Source: CAD feature listing. Evaluate the final solid. Frame: model axes, mm. Face numbers are marked on the shaded views. A direction names the side the tool comes from. Coordinates: 2 decimals unless noted, no trailing zeros. Write each loop counter-clockwise with the first axis right and the second up, starting at its lowest first coordinate (ties: lowest second). Pieces come first, ordered by that corner, then holes. Notation, with made-up numbers: M 83.5,0 L 126.5,0 A17 ccw 126.5,12 Z; hole C 74.25,-19.75 d2. An arc over 180 degrees is marked long. One line per item, written item: value. Start each with the question number.
Item 1: Cut plane A-A, the plane z = -98.5. Output: boundary loops of the cut face in (x, y), then the cut area to 3 significant figures.
Item 2: Ray query, L1, parallel to X at y = 19.5, z = -37; L2, parallel to Z at x = 19, y = 0.5; L3, parallel to Z at x = 75.5, y = -14. Return the intervals inside material, ascending. Write a range as from..to.
Item 3: Cut plane B-B, the plane y = 0. Output: boundary loops of the cut face in (x, z), then the cut area to 3 significant figures.
Item 4: Cut plane D-D, the plane z = 0. Output: boundary loops of the cut face in (x, y).
Item 5: Cut plane C-C, the plane x = 140.5. Output: boundary loops of the cut face in (y, z), then the cut area to 3 significant figures.
Item 6: Mould query, pull axis X, two halves, no side actions, for the marked faces 1, 2 and 3. Classes: released by +X, released by -X, zero draft, split by the parting line, or undercut.
Item 7: Set-up query: the marked faces 4, 5, 6, 7 and 8. Return all of +Z, -Z, +X, -X, +Y, -Y with unobstructed straight access to the full face (end or side cutting, diameter ignored); none if empty.
Item 8: Pin query (flat end, axial travel): P1, Ø12, axis at y = -7, z = -57, coming from the +X side; P2, Ø4.5, axis at y = -5, z = -223, coming from the +X side; P3, Ø10, axis at x = -26, z = -142, coming from the -Y side. Return the tip coordinate at first contact, or that it passes through.
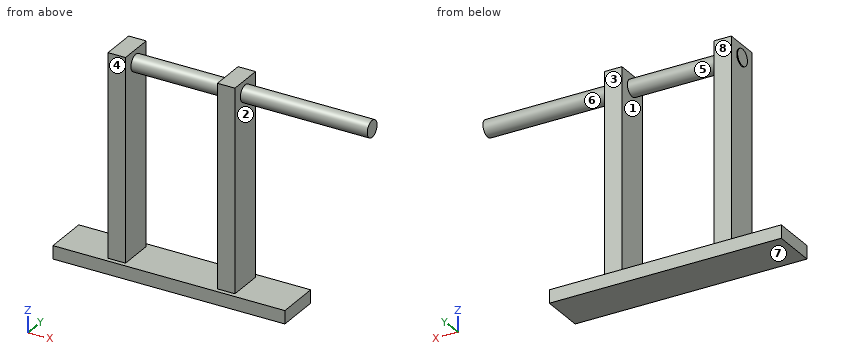
```python
from build123d import *

# Parameters (mm, degrees)
F0_R      = 9.5
F1_DEPTH  = 40
F2_R      = 9.5
F3_DEPTH  = 70
F4_R      = 9.5
F5_DEPTH  = 180
F6_W      = 20
F6_H      = 20
F7_DEPTH  = 15
F8_W      = 20
F8_H      = 10
F9_DEPTH  = 215
F11_DEPTH = 15
F12_DEPTH = 15
F13_DEPTH = 215
F15_DEPTH = 215
F16_W     = 20
F16_H     = 7.5
F17_DEPTH = 20
F18_DEPTH = 25
F19_DEPTH = 25
F20_R     = 9.5
F21_DEPTH = 1


with BuildPart() as f1:
    # F0 (on Right) → F1 (new body)
    with BuildSketch(Plane.YZ):
        Circle(F0_R)
    extrude(amount=-F1_DEPTH)

    # F2 (on face) → F3 (join)
    with BuildSketch(Plane.YZ):
        Circle(F2_R)
    extrude(amount=F3_DEPTH)

    # F4 (on face) → F5 (join)
    with BuildSketch(Plane.YZ.offset(70)):
        Circle(F4_R)
    extrude(amount=F5_DEPTH)

    # F6 (on Top) → F7 (join)
    with BuildSketch(Plane.XY):
        with Locations((-30, -10)):
            Rectangle(F6_W, F6_H)
        with Locations((-30, 10)):
            Rectangle(F6_W, F6_H)
    extrude(amount=F7_DEPTH)

    # F8 (on Top) → F9 (join)
    with BuildSketch(Plane.XY):
        with Locations((-30, -5)):
            Rectangle(F8_W, F8_H)
        with Locations((-30, 5)):
            Rectangle(F8_W, F8_H)
        with Locations((-30, -15)):
            Rectangle(F8_W, F8_H)
        with Locations((-30, 15)):
            Rectangle(F8_W, F8_H)
    extrude(amount=-F9_DEPTH)

    # F10 (on Top) → F11 (join)
    with BuildSketch(Plane.XY):
        Polygon((85, 10), (85, 0), (85, -10), (85, -20), (105, -20), (105, 20), (85, 20), align=None)
    extrude(amount=F11_DEPTH)

    # F6 (on Top) → F12 (join)
    with BuildSketch(Plane.XY):
        with Locations((-30, -10)):
            Rectangle(F6_W, F6_H)
        with Locations((-30, 10)):
            Rectangle(F6_W, F6_H)
    extrude(amount=F12_DEPTH)

    # F8 (on Top) → F13 (join)
    with BuildSketch(Plane.XY):
        with Locations((-30, -5)):
            Rectangle(F8_W, F8_H)
        with Locations((-30, 5)):
            Rectangle(F8_W, F8_H)
        with Locations((-30, -15)):
            Rectangle(F8_W, F8_H)
        with Locations((-30, 15)):
            Rectangle(F8_W, F8_H)
    extrude(amount=-F13_DEPTH)

    # F14 (on Top) → F15 (join)
    with BuildSketch(Plane.XY):
        Polygon((85, 20), (85, 0), (85, -20), (105, -20), (105, 20), align=None)
    extrude(amount=-F15_DEPTH)

    # F16 (on Front) → F17 (join)
    with BuildSketch(Plane.XZ):
        with Locations((-30, -218.75)):
            Rectangle(F16_W, F16_H)
    extrude(amount=F17_DEPTH)

    # F16 (on Front) → F18 (join)
    with BuildSketch(Plane.XZ):
        Polygon((85, -215), (0, -215), (-20, -215), (-20, -222.5), (85, -222.5), align=None)
        with Locations((-30, -218.75)):
            Rectangle(F16_W, F16_H)
        with Locations((95, -218.75)):
            Rectangle(F16_W, F16_H)
        Polygon((-40, -222.5), (-40, -215), (-100, -215), (-100, -230), (-40, -230), align=None)
        Polygon((85, -222.5), (-20, -222.5), (-40, -222.5), (-40, -230), (165, -230), (165, -215), (105, -215), (105, -222.5), align=None)
    extrude(amount=F18_DEPTH)

    # F16 (on Front) → F19 (join)
    with BuildSketch(Plane.XZ):
        Polygon((85, -215), (0, -215), (-20, -215), (-20, -222.5), (85, -222.5), align=None)
        with Locations((-30, -218.75)):
            Rectangle(F16_W, F16_H)
        with Locations((95, -218.75)):
            Rectangle(F16_W, F16_H)
        Polygon((-40, -222.5), (-40, -215), (-100, -215), (-100, -230), (-40, -230), align=None)
        Polygon((85, -222.5), (-20, -222.5), (-40, -222.5), (-40, -230), (165, -230), (165, -215), (105, -215), (105, -222.5), align=None)
    extrude(amount=-F19_DEPTH)

    # F20 (on face) → F21 (join)
    with BuildSketch(Plane(origin=(-40, 0, 0), x_dir=(0, -1, 0), z_dir=(-1, 0, 0))):
        Circle(F20_R)
    extrude(amount=F21_DEPTH)


solid = f1.part
```
From the geometry:
1. outline: M -40,-20 L -20,-20 L -20,20 L -40,20 Z; M 85,-20 L 105,-20 L 105,20 L 85,20 Z
1. area: 1,600 mm²
2. L1: x = -40..-20, 85..105
2. L2: z = -230..-215, -9.49..9.49
2. L3: z = -230..-215
3. outline: M -100,-230 L 165,-230 L 165,-215 L 105,-215 L 105,-9.5 L 250,-9.5 L 250,9.5 L 105,9.5 L 105,15 L 85,15 L 85,9.5 L -20,9.5 L -20,15 L -40,15 L -40,9.5 L -41,9.5 L -41,-9.5 L -40,-9.5 L -40,-215 L -100,-215 Z; hole M -20,-215 L 85,-215 L 85,-9.5 L -20,-9.5 Z
3. area: 17,900 mm²
4. outline: M -41,-9.5 L -40,-9.5 L -40,-20 L -20,-20 L -20,-9.5 L 85,-9.5 L 85,-20 L 105,-20 L 105,-9.5 L 250,-9.5 L 250,9.5 L 105,9.5 L 105,20 L 85,20 L 85,9.5 L -20,9.5 L -20,20 L -40,20 L -40,9.5 L -41,9.5 Z
5. outline: M -25,-230 L 25,-230 L 25,-215 L -25,-215 Z; C 0,0 d19
5. area: 1,030 mm²
6. face 1: undercut
6. face 2: released by +X
6. face 3: zero draft
7. face 4: +Z, +X, -X, -Y
7. face 5: none
7. face 6: +X
7. face 7: -Z, +X, -X, +Y, -Y
7. face 8: +Z, +X, -X, +Y
8. P1: stops at x = 105
8. P2: stops at x = 165
8. P3: stops at y = -20
